Check sheet for the drawn part. Datum: minimum x, y, z corner. Units: mm. Give positions to 0.01 mm unless a question says otherwise; leave off trailing zeros. Write each loop counter-clockwise with the first axis right and the second up, starting at its lowest first coordinate (ties: lowest second). Pieces come first, ordered by that corner, then holes. Notation, with made-up numbers: M 9.5,69.25 L 37.5,69.25 A31 cw 37.5,108.25 Z; hole C -37,-7 d1. An arc over 180 degrees is marked long. Write item = value, one per line. Start each with the question number.
1) Scan line: L1, parallel to X at y = 2.9, z = 30 (3 decimals). Record every from-to range of solid material in increasing order.
2) Sectioned sample at A-A, the plane y = 2.6. Record the cut outline in (x, z) (3 decimals).
3) Gauge pin test, flat ends, axial feed: pin 1 (1 mm diameter, centred on y = 1.5, z = 29.5, fed in from -X) (3 decimals); pin 2 (1 mm diameter, centred on x = 62, y = 2, fed in from -Z); pin 3 (1.6 mm diameter, centred on y = 2.5, z = 3.5, fed in from +X) (3 decimals). Record the tip position at first contact, or that the pin passes through.
4) Sectioned sample at B-B, the plane z = 61. Record the cut outline in (x, y) (3 decimals).
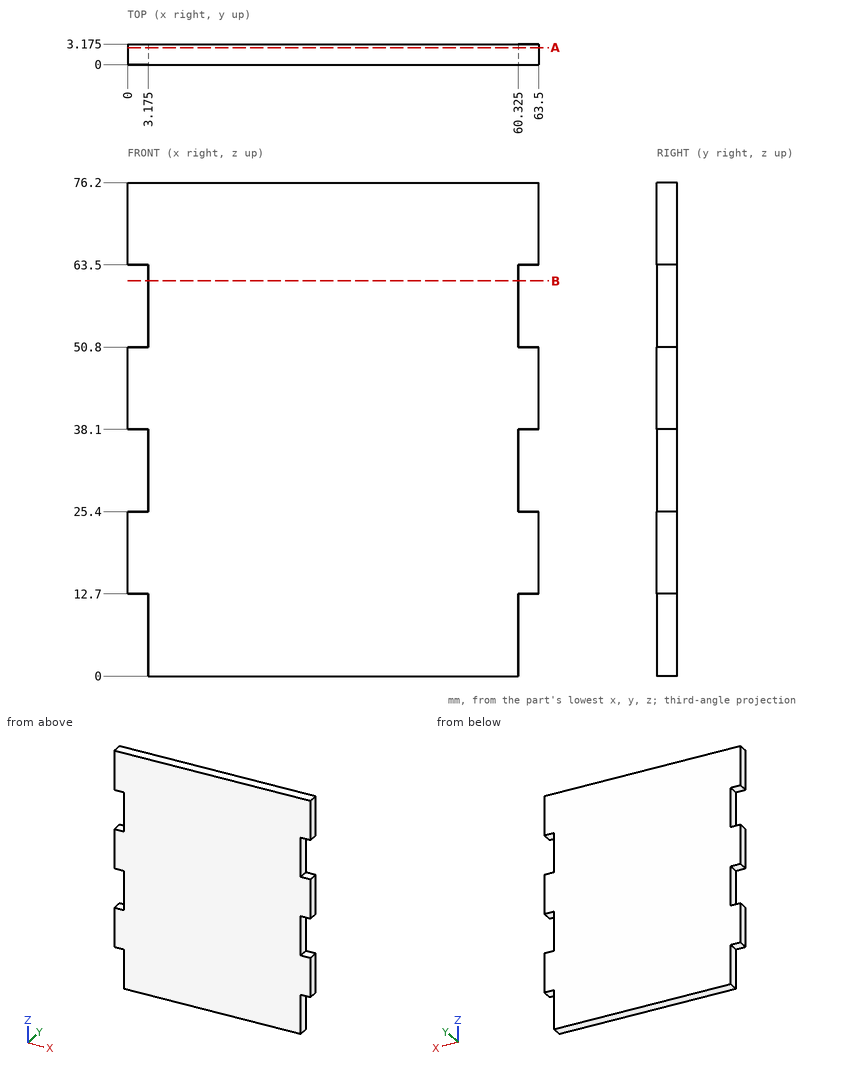
Data:
q1.L1 = 3.175 to 60.325
q2.outline = M 0,12.7 L 3.175,12.7 L 3.175,0 L 60.325,0 L 60.325,12.7 L 63.5,12.7 L 63.5,25.4 L 60.325,25.4 L 60.325,38.1 L 63.5,38.1 L 63.5,50.8 L 60.325,50.8 L 60.325,63.5 L 63.5,63.5 L 63.5,76.2 L 0,76.2 L 0,63.5 L 3.175,63.5 L 3.175,50.8 L 0,50.8 L 0,38.1 L 3.175,38.1 L 3.175,25.4 L 0,25.4 Z
q3.pin_1 = 3.175
q3.pin_2 = 12.7
q3.pin_3 = 60.325
q4.outline = M 3.175,0 L 60.325,0 L 60.325,3.175 L 3.175,3.175 Z
